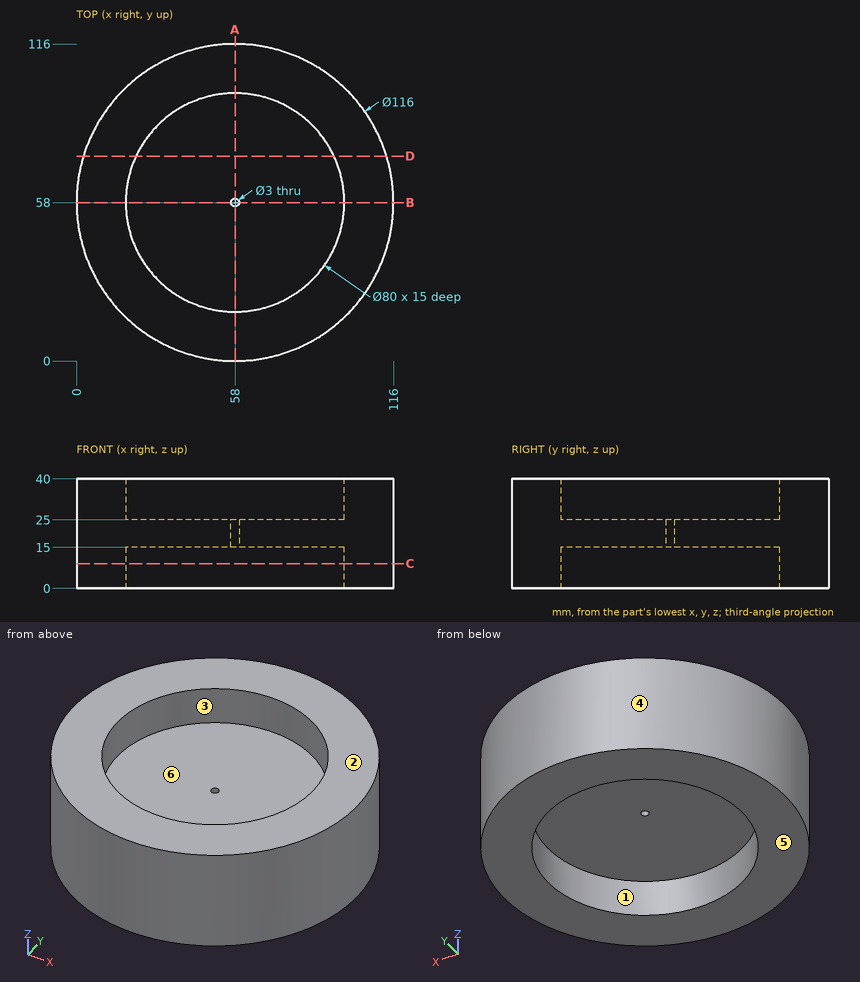
For this review, use the dimensioned drawing (mm, ordinates from the lowest corner) and the shaded views. A direction names the side the tool comes from. Round coordinates to 2 decimals unless told otherwise and drop trailing zeros. Order: outer loops, then holes, each group sorted by start corner. A loop starts at its lowest first (then second) coordinate and runs counter-clockwise, first axis right, second up.
1) Consider section D-D (y = 75). State the section outline as (x, z) points.
The answers:
outline: (2.55, 0) - (21.79, 0) - (21.79, 15) - (94.21, 15) - (94.21, 0) - (113.45, 0) - (113.45, 40) - (94.21, 40) - (94.21, 25) - (21.79, 25) - (21.79, 40) - (2.55, 40) - close
2) Consider section A-A (x = 58). State the section outline as (y, z) points.
The answers:
outline: (0, 0) - (18, 0) - (18, 15) - (56.5, 15) - (56.5, 25) - (18, 25) - (18, 40) - (0, 40) - close; (59.5, 15) - (98, 15) - (98, 0) - (116, 0) - (116, 40) - (98, 40) - (98, 25) - (59.5, 25) - close
3) Consider section C-C (z = 9). State the section outline as (x, y) points, plus the area to 3 significant figures.
The answers:
outline: circle Ø116 at (58, 58); hole circle Ø80 at (58, 58)
area: 5,540 mm2
4) Clearance check with flat-ended pins moving along their axes: pin 1 Ø8 at (x, z) = (98, 12) entering from -Y; pin 2 Ø5 at (y, z) = (13, 8.5) entering from +X; pin 3 Ø12 at (y, z) = (82.5, 26) entering from -X. State where each tip first meets the part, or that it passes through.
The answers:
pin 1: stops at y = 12.52
pin 2: stops at x = 97.47
pin 3: stops at x = 3.03
5) For L1, parallel to Z at x = 38, y = 49; L2, parallel to Y at x = 72.5, z = 26.5; L3, parallel to Y at x = 84.5, z = 4, list the stretches that pass through material, from the lowest coordinate up.
The answers:
L1: z = 15 to 25
L2: y = 1.84 to 20.72, 95.28 to 114.16
L3: y = 6.41 to 28.04, 87.96 to 109.59
6) Machinability: for the marked faces 1 and 2, which of the approach directions +Z, -Z, +X, -X, +Y, -Y give a long, thin tool a straight path to every point of the face, cutting with its end or side? Answer none if there is none.
The answers:
face 1: -Z
face 2: +Z, +X, -X, +Y, -Y
7) Draft analysis for pull direction Y (two halves, no side actions). For the marked faces 3, 4, 5 and 6, state which applies: released by +Y, released by -Y, zero draft, split by the parting line, or undercut.
The answers:
face 3: undercut
face 4: split by the parting line
face 5: zero draft
face 6: undercut
